Work out the finished part from the listing and answer in its coordinate system (mm). A direction names the side the tool comes from. Give positions to 0.01 mm unless a question says otherwise; leave off trailing zeros. Loops run counter-clockwise (first coordinate to the right, second up) from the corner with the lowest first, then second, coordinate; pieces in that order, holes last. Notation, with made-up numbers: M 23,49 L 51,49 A15 ccw 51,74 Z; hole C -32.5,-29.5 d10. An arc over 180 degrees is marked long. Answer in a Markdown table with one row per item. Add a question column.
Autodesk Inventor part; units mm, degrees
ref_plane "YZ Plane" through (0, 0, 0) normal (1, 0, 0) x (0, 1, 0)
ref_plane "XZ Plane" through (0, 0, 0) normal (0, 1, 0) x (-1, 0, 0)
ref_plane "XY Plane" through (0, 0, 0) normal (0, 0, 1) x (1, 0, 0)
sketch "Эскиз1" plane through (0, 0, 0) normal (0, 0, 1) x (1, 0, 0)
  line L0 (0, 0) -> (0, 60) construction
  line L1 (0, 60) -> (-15, 60)
  line L2 (-15, 60) -> (-15, 64)
  line L3 (-15, 64) -> (-35, 64)
  line L4 (-35, 64) -> (-35, 60)
  line L5 (-35, 60) -> (-49, 60)
  line L6 (-49, 60) -> (-49, 45)
  line L7 (-49, 45) -> (-53, 45)
  line L8 (-53, 45) -> (-53, 15)
  line L9 (-53, 15) -> (-49, 15)
  line L10 (-49, 15) -> (-49, 0)
  line L11 (-49, 0) -> (-35, 0)
  line L12 (-35, 0) -> (-35, -4)
  line L13 (-35, -4) -> (-15, -4)
  line L14 (-15, -4) -> (-15, 0)
  line L15 (-15, 0) -> (0, 0)
  line L16 (0, 60) -> (15, 60)
  line L17 (15, 60) -> (15, 64)
  line L18 (15, 64) -> (35, 64)
  line L19 (35, 64) -> (35, 60)
  line L20 (35, 60) -> (49, 60)
  line L21 (49, 60) -> (49, 45)
  line L22 (49, 45) -> (53, 45)
  line L23 (53, 45) -> (53, 15)
  line L24 (53, 15) -> (49, 15)
  line L25 (49, 15) -> (49, 0)
  line L26 (49, 0) -> (35, 0)
  line L27 (35, 0) -> (35, -4)
  line L28 (35, -4) -> (15, -4)
  line L29 (15, -4) -> (15, 0)
  line L30 (15, 0) -> (0, 0)
  line L31 (-39, 50) -> (39, 50)
  line L32 (39, 50) -> (39, 10)
  line L33 (39, 10) -> (-39, 10)
  line L34 (-39, 10) -> (-39, 50)
  point P0 (-53, 30)
  point P1 (0, 30)
  point P2 (53, 30)
  dimension "d0" = 30
  dimension "d1" = 4
  dimension "d2" = 98
  dimension "d3" = 30
  dimension "d4" = 20
  dimension "d5" = 60
  dimension "d6" = 10
  dimension "d7" = 10
  dimension "d8" = 10
extrude "Выдавливание1" add sketch "Эскиз1" along normal blind 4
fillet "Сопряжение1" radius 8 4 edges at (-39, 10, 2) (-39, 50, 2) (39, 50, 2) (39, 10, 2)
sketch "Эскиз2" plane through (0, 0, 4) normal (0, 0, 1) x (1, 0, 0)
  line L0 (0, 0) -> (0, 60)
  line L1 (-15, 60) -> (15, 60)
  line L2 (-35, 60) -> (-49, 60)
  line L3 (-49, 0) -> (-35, 0)
  line L4 (-49, 60) -> (-49, 45)
  point P0 (44, 10)
  point P1 (44, 50)
  point P2 (-44, 10)
  point P3 (-44, 50)
  dimension "d19" = 10
  dimension "d20" = 10
  dimension "d21" = 5
hole "Отверстие1" at (44, 10, 4) at (44, 50, 4) at (-44, 10, 4) at (-44, 50, 4) direction (0, 0, -1) diameter 3 end through all
properties part number "stiffenerFront" material "Дерево (береза)"
(1) Each of these flat-tipped pins is pushed along its axis until it touches: P1, Ø1, axis at x = -5.5, z = 2, coming from the -Y side; P2, Ø1.2, axis at y = 55.5, z = 2.5, coming from the +X side; P3, Ø1.8, axis at x = 44, y = 50, coming from the -Z side. Where does it stop, or does it pass through?
(2) Consider line 1 along Y through (x, z) = (-44, 2.9); line 2 along Y through (x, z) = (12, 3); line 3 along Y through (x, z) = (27, 2.75). Determine where each line is inside the solid, lowest interval first. Write a range as from..to.
(3) Section A-A, the plane x = 44 is taken. Determine the outline of the cut face in (y, z).
(4) Section D-D, the plane z = 2.75 is taken. State how many separate pieces and enclosed holes the cut face has, and give its area (3 significant figures).
(5) The mould has two halves that part along Y. Classify faces 4 (the face through (-42, 60, 2)), 5 (the face through (-1, 8, 0)), 6 (the face through (0, 10, 2)), 7 (the face through (-42.536, 10.325, 1.972)): pulls with the +Y half, pulls with the -Y half, needs draft (parallel to the pull), parting line crosses it, or undercut.
(6) Section C-C, the plane x = 21.5 is taken. Determine the outline of the cut face in (y, z), and give its area (3 significant figures).
(7) Section B-B, the plane y = 29 is taken. Determine the outline of the cut face in (x, z), and give its area (3 significant figures).
(8) Which of the six approach directions +Z, -Z, +X, -X, +Y, -Y give full straight-line access (tool end or side, diameter ignored) to faces 1 (the face through (-49, 53, 2)), 2 (the face through (49, 8, 2)), 3 (the face through (0, 60, 2))?
Numbers:
| question | item | result |
|---|---|---|
| 1 | P1 | stops at y = 0 |
| 1 | P2 | stops at x = 49 |
| 1 | P3 | passes through |
| 2 | line 1 | y = 0..8.5, 11.5..48.5, 51.5..60 |
| 2 | line 2 | y = 0..10, 50..60 |
| 2 | line 3 | y = -4..10, 50..64 |
| 3 | outline | M 0,0 L 8.5,0 L 8.5,4 L 0,4 Z; M 11.5,0 L 48.5,0 L 48.5,4 L 11.5,4 Z; M 51.5,0 L 60,0 L 60,4 L 51.5,4 Z |
| 4 | separate pieces | 1 |
| 4 | enclosed holes | 5 |
| 4 | area | 3,350 mm² |
| 5 | face 4 | pulls with the +Y half |
| 5 | face 5 | needs draft |
| 5 | face 6 | undercut |
| 5 | face 7 | undercut |
| 6 | outline | M -4,0 L 10,0 L 10,4 L -4,4 Z; M 50,0 L 64,0 L 64,4 L 50,4 Z |
| 6 | area | 112 mm² |
| 7 | outline | M -53,0 L -39,0 L -39,4 L -53,4 Z; M 39,0 L 53,0 L 53,4 L 39,4 Z |
| 7 | area | 112 mm² |
| 8 | face 1 | +Z, -Z, -X, +Y |
| 8 | face 2 | +Z, -Z, +X, -Y |
| 8 | face 3 | +Z, -Z, +Y |
